For this review, take the finished solid that the model builds, in its own axes (mm). A direction names the side the tool comes from. Coordinates: 2 decimals unless noted, no trailing zeros. Write each loop counter-clockwise with the first axis right and the second up, starting at its lowest first coordinate (ties: lowest second). Pieces come first, ordered by that corner, then holes. Notation, with made-up numbers: (83.25, 86) - (92.25, 86) arc R17 cw to (92.25, 111) - close; hole circle Ø3 at (17.25, 41.5). An arc over 180 degrees is marked (long way). Write each question's results on one line, items separated by ' | '.
from build123d import *

# Parameters (mm, degrees)
SKETCH1_W           = 130
SKETCH1_H           = 145.26
SKETCH1_R           = 3.6
SKETCH1_R_2         = 2.5
BOSS_EXTRUDE1_DEPTH = 9.4
SKETCH2_R           = 2.5
CUT_EXTRUDE1_DEPTH  = 10.4
CUT_EXTRUDE2_DEPTH  = 10.4
CUT_EXTRUDE3_DEPTH  = 10.4
SKETCH5_R           = 2.5
CUT_EXTRUDE4_DEPTH  = 10.4


with BuildPart() as part:
    # Sketch1 → Boss-Extrude1 (new body)
    with BuildSketch(Plane.XY):
        with Locations((50, 62.63)):
            Rectangle(SKETCH1_W, SKETCH1_H)
        Circle(SKETCH1_R, mode=Mode.SUBTRACT)
        with Locations((0, 60.26)):
            Circle(SKETCH1_R_2, mode=Mode.SUBTRACT)
        with Locations((100, 60.26)):
            Circle(SKETCH1_R_2, mode=Mode.SUBTRACT)
        with Locations((100, 0)):
            Circle(SKETCH1_R, mode=Mode.SUBTRACT)
    extrude(amount=BOSS_EXTRUDE1_DEPTH)

    # Sketch2 → Cut-Extrude1 (cut, through all)
    with BuildSketch(Plane.XY.offset(9.4)):
        with Locations((75.33, 122.766411568)):
            Circle(SKETCH2_R)
        with Locations((75.33, 102.766411568)):
            Circle(SKETCH2_R)
    extrude(amount=-CUT_EXTRUDE1_DEPTH, mode=Mode.SUBTRACT)

    # Sketch3 → Cut-Extrude2 (cut, through all)
    with BuildSketch(Plane(origin=(0, 0, 0), x_dir=(-1, 0, 0), z_dir=(0, 0, -1))):
        with BuildLine():
            Line((-35.40754614, 117.570367495), (-30.40754614, 117.570367495))
            ThreePointArc((-30.40754614, 117.570367495), (-26.872012234, 116.105901401), (-25.40754614, 112.570367495))
            Line((-25.40754614, 112.570367495), (-25.40754614, 92.570367495))
            ThreePointArc((-25.40754614, 92.570367495), (-26.872012234, 89.034833589), (-30.40754614, 87.570367495))
            Line((-30.40754614, 87.570367495), (-35.40754614, 87.570367495))
            ThreePointArc((-35.40754614, 87.570367495), (-38.943080046, 89.034833589), (-40.40754614, 92.570367495))
            Line((-40.40754614, 92.570367495), (-40.40754614, 112.570367495))
            ThreePointArc((-40.40754614, 112.570367495), (-38.943080046, 116.105901401), (-35.40754614, 117.570367495))
        make_face()
    extrude(amount=-CUT_EXTRUDE2_DEPTH, mode=Mode.SUBTRACT)

    # Sketch4 → Cut-Extrude3 (cut, through all)
    with BuildSketch(Plane.XY.offset(9.4)):
        with BuildLine():
            Line((-15, 78.5), (-15, 94.86))
            Line((-15, 94.86), (-0.81, 94.86))
            ThreePointArc((-0.81, 94.86), (7.37, 86.68), (-0.81, 78.5))
            Line((-0.81, 78.5), (-15, 78.5))
        make_face()
    extrude(amount=-CUT_EXTRUDE3_DEPTH, mode=Mode.SUBTRACT)

    # Sketch5 → Cut-Extrude4 (cut, through all)
    with BuildSketch(Plane.XY.offset(9.4)):
        with Locations((-4.926856844, 105.186)):
            Circle(SKETCH5_R)
        with Locations((15.215343156, 105.186)):
            Circle(SKETCH5_R)
    extrude(amount=-CUT_EXTRUDE4_DEPTH, mode=Mode.SUBTRACT)


solid = part.part
Q1. Take a section at C-C on z = 2.25. State how many separate pieces and enclosed holes the cut face has, plus the area to 3 significant figures.
Results found:
separate pieces: 1 | enclosed holes: 9 | area: 17,900 mm2
Q2. Mouldability with a two-part tool opening along Y and no side actions: class faces 4 (the face through (-0.33, 62.74, 4.63)), 5 (the face through (49, 135.26, 5)), 6 (the face through (115, 62, 5)) as pulls with the +Y half, pulls with the -Y half, needs draft (parallel to the pull), parting line crosses it, or undercut.
Results found:
face 4: undercut | face 5: pulls with the +Y half | face 6: needs draft
Q3. Take a section at B-B on y = 60.26. State the section outline as (x, z) points, plus the area to 3 significant figures.
Results found:
outline: (-15, 0) - (-2.5, 0) - (-2.5, 9.4) - (-15, 9.4) - close; (2.5, 0) - (97.5, 0) - (97.5, 9.4) - (2.5, 9.4) - close; (102.5, 0) - (115, 0) - (115, 9.4) - (102.5, 9.4) - close | area: 1,130 mm2
Q4. Wall thickness on line 1 along Y through (x, z) = (-5, 7.5); line 2 along Y through (x, z) = (100, 2.25); line 3 along X through (y, z) = (123, 2.5): over which ranges is each line inside the solid? List them lowest first. Write a range as from..to.
Results found:
line 1: -10..78.5, 94.86..102.69, 107.68..135.26 | line 2: -10..-3.6, 3.6..57.76, 62.76..135.26 | line 3: -15..72.84, 77.82..115
Q5. Take a section at A-A on x = 75.33. State the section outline as (y, z) points, plus the area to 3 significant figures.
Results found:
outline: (-10, 0) - (100.27, 0) - (100.27, 9.4) - (-10, 9.4) - close; (105.27, 0) - (120.27, 0) - (120.27, 9.4) - (105.27, 9.4) - close; (125.27, 0) - (135.26, 0) - (135.26, 9.4) - (125.27, 9.4) - close | area: 1,270 mm2
Q6. For faces 1 (the face through (25.408, 103, 5)), 2 (the face through (49, -10, 5)), 3 (the face through (-8, 94.86, 5)), list the 3-axis set-ups (+Z, -Z, +X, -X, +Y, -Y) from which the entire face can be reached by the end or side of a thin tool; tool diameter is ignored.
Results found:
face 1: +Z, -Z | face 2: +Z, -Z, +X, -X, -Y | face 3: +Z, -Z, -X
